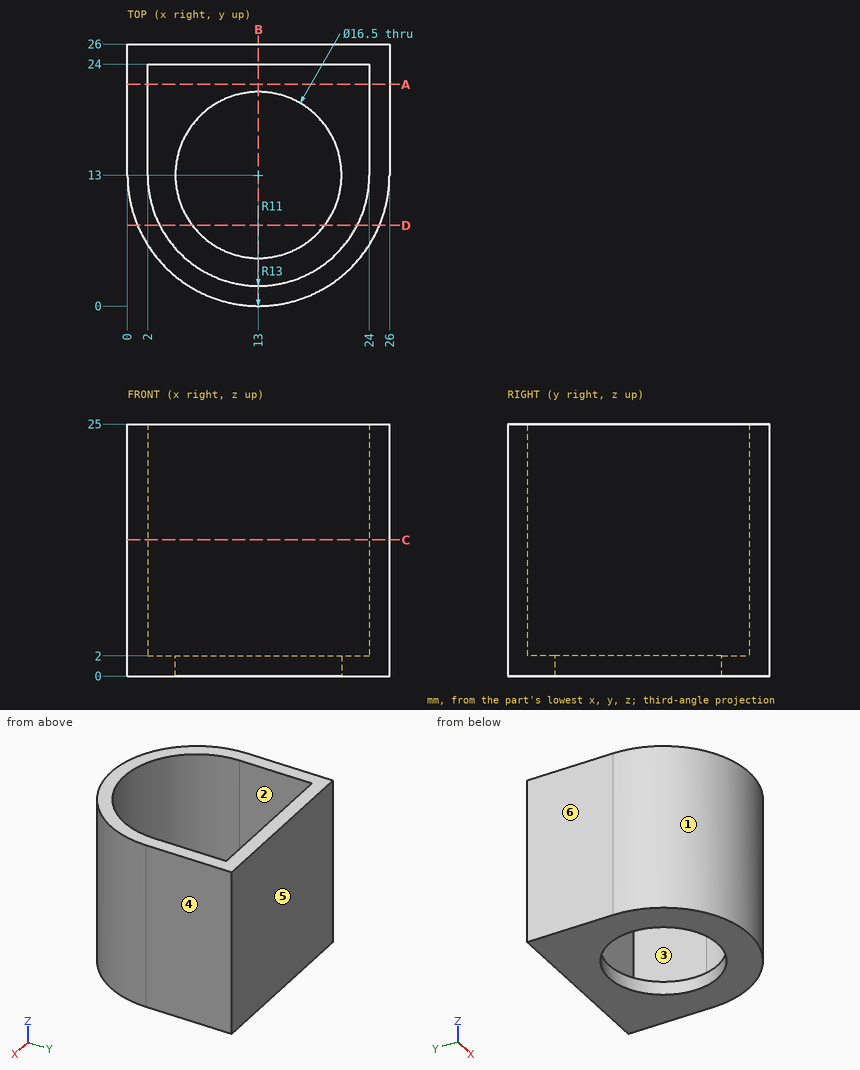
Drawing for the job (mm, zero at the part's lowest x, y, z). A direction names the side the tool comes from. Give positions to 0.01 mm unless a question says otherwise; leave off trailing zeros. Order: outer loops, then holes, each group sorted by start corner. A loop starts at its lowest first (then second) coordinate and runs counter-clockwise, first axis right, second up. Notation, with made-up numbers: (73.25, 21) -> (105.25, 21) arc R11 ccw to (105.25, 36) -> close; hole circle Ø11 at (-33, 5.25). An arc over 180 degrees is marked (long way). Use one line per item in the form item = value.
(1) Flat gauge pins, fed straight in: P1, Ø5, axis at y = 17.5, z = 8.5, coming from the -X side; P2, Ø10, axis at x = 5, z = 21.5, coming from the -Y side; P3, Ø6, axis at y = 7, z = 13, coming from the +X side. Where does each tip first touch, or does it go through?
Solution:
P1 = 0
P2 = 0.35
P3 = 25.65
(2) Pull direction X, two halves, no side cores. Call the marked faces 3, 4, 5 and 6: +X half, -X half, draft (parallel to the pull), parting line (faces both ways), or undercut.
Solution:
face_3 = undercut
face_4 = +X half
face_5 = draft
face_6 = -X half
(3) Saw through at C-C (z = 13.5). Write the cut outline in (x, y), then the cut area to 3 significant figures.
Solution:
outline = (0, 13) arc R13 ccw to (26, 13) -> (26, 26) -> (0, 26) -> close; hole (2, 13) arc R11 ccw to (24, 13) -> (24, 24) -> (2, 24) -> close
area = 171 mm²
(4) Saw through at B-B (x = 13). Write the cut outline in (y, z), then the cut area to 3 significant figures.
Solution:
outline = (0, 0) -> (4.75, 0) -> (4.75, 2) -> (2, 2) -> (2, 25) -> (0, 25) -> close; (21.25, 0) -> (26, 0) -> (26, 25) -> (24, 25) -> (24, 2) -> (21.25, 2) -> close
area = 111 mm²
(5) Tool access for the marked faces 1 and 2: list every direction of +Z, -Z, +X, -X, +Y, -Y with a clear straight run to the whole face (end or side of a thin tool).
Solution:
face_1 = +Z, -Z, -Y
face_2 = +Z
(6) Saw through at D-D (y = 8). Write the cut outline in (x, z).
Solution:
outline = (1, 0) -> (6.44, 0) -> (6.44, 2) -> (3.2, 2) -> (3.2, 25) -> (1, 25) -> close; (19.56, 0) -> (25, 0) -> (25, 25) -> (22.8, 25) -> (22.8, 2) -> (19.56, 2) -> close
(7) Drill centre lines: line 1 (X direction, y = 13.75, z = 4.75); line 2 (Y direction, x = 13, z = 1.2). Where is each one in solid material? Low to high. Write a range as from..to.
Solution:
line_1 = 0..2, 24..26
line_2 = 0..4.75, 21.25..26
(8) Saw through at A-A (y = 22). Write the cut outline in (x, z).
Solution:
outline = (0, 0) -> (26, 0) -> (26, 25) -> (24, 25) -> (24, 2) -> (2, 2) -> (2, 25) -> (0, 25) -> close
